from build123d import *

# Parameters (mm, degrees)
F1_DEPTH = 6.35


with BuildPart() as f1:
    # F0 (on Top) → F1 (new body)
    with BuildSketch(Plane.XY):
        with BuildLine():
            ThreePointArc((-3.1267646158, 0.5513329641), (0.2767194832, 3.1629181664), (3.175, 0))
            Line((3.175, 0), (9.525, 0))
            ThreePointArc((9.525, 0), (6.7351920908, 6.7351920908), (0, 9.525))
            ThreePointArc((0, 9.525), (-6.1225519823, 7.2965733207), (-9.3802938474, 1.6539988923))
            Line((-9.3802938474, 1.6539988923), (-3.1267646158, 0.5513329641))
        make_face()
        with BuildLine():
            Line((9.525, 0), (3.175, 0))
            ThreePointArc((3.175, 0), (0, -3.175), (-3.175, 0))
            Line((-3.175, 0), (-9.525, 0))
            ThreePointArc((-9.525, 0), (-7.8202053152, -5.4378317212), (-3.316073212, -8.9291255704))
            Line((-3.316073212, -8.9291255704), (0, -9.525))
            ThreePointArc((0, -9.525), (6.7351920908, -6.7351920908), (9.525, 0))
        make_face()
        with BuildLine():
            ThreePointArc((0, 9.525), (6.7351920908, 6.7351920908), (9.525, 0))
            Line((9.525, 0), (50.1904, 0))
            ThreePointArc((50.1904, 0), (52.9802079092, 6.7351920908), (59.7154, 9.525))
            Line((59.7154, 9.525), (0, 9.525))
        make_face()
        with BuildLine():
            Line((50.1904, 0), (9.525, 0))
            ThreePointArc((9.525, 0), (6.7351920908, -6.7351920908), (0, -9.525))
            Line((0, -9.525), (59.7154, -9.525))
            ThreePointArc((59.7154, -9.525), (52.9802079092, -6.7351920908), (50.1904, 0))
        make_face()
        with BuildLine():
            ThreePointArc((-3.316073212, -8.9291255704), (-7.8202053152, -5.4378317212), (-9.525, 0))
            Line((-9.525, 0), (-40.1437268637, 0))
            ThreePointArc((-40.1437268637, 0), (-42.2877419599, -1.0354554234), (-44.6215756209, -1.5068248214))
            Line((-44.6215756209, -1.5068248214), (-3.316073212, -8.9291255704))
        make_face()
        with BuildLine():
            Line((-35.9452860234, 6.3381237552), (-9.3802938474, 1.6539988923))
            ThreePointArc((-9.3802938474, 1.6539988923), (-6.1225519823, 7.2965733207), (0, 9.525))
            Line((0, 9.525), (-43.6409873472, 17.3669705411))
            ThreePointArc((-43.6409873472, 17.3669705411), (-38.0190290845, 14.1027642346), (-35.8005798708, 7.9921226475))
            ThreePointArc((-35.8005798708, 7.9921226475), (-35.8368253715, 7.1619641978), (-35.9452860234, 6.3381237552))
        make_face()
        with BuildLine():
            ThreePointArc((59.7154, 9.525), (52.9802079092, 6.7351920908), (50.1904, 0))
            ThreePointArc((50.1904, 0), (52.9802079092, -6.7351920908), (59.7154, -9.525))
            ThreePointArc((59.7154, -9.525), (66.4505920908, -6.7351920908), (69.2404, 0))
            ThreePointArc((69.2404, 0), (66.4505920908, 6.7351920908), (59.7154, 9.525))
        make_face()
        with BuildLine():
            ThreePointArc((62.8904, 0), (59.7154, -3.175), (56.5404, 0))
            ThreePointArc((56.5404, 0), (59.7154, 3.175), (62.8904, 0))
        make_face(mode=Mode.SUBTRACT)
        with BuildLine():
            ThreePointArc((-3.316073212, -8.9291255704), (-1.6845925237, -9.3748478937), (0, -9.525))
            Line((0, -9.525), (-3.316073212, -8.9291255704))
        make_face()
        with BuildLine():
            ThreePointArc((-44.6215756209, -1.5068248214), (-42.2877419599, -1.0354554234), (-40.1437268637, 0))
            ThreePointArc((-40.1437268637, 0), (-37.3847371298, 2.7320236406), (-35.9452860234, 6.3381237552))
            ThreePointArc((-35.9452860234, 6.3381237552), (-35.8368253715, 7.1619641978), (-35.8005798708, 7.9921226475))
            ThreePointArc((-35.8005798708, 7.9921226475), (-38.0190290845, 14.1027642346), (-43.6409873472, 17.3669705411))
            ThreePointArc((-43.6409873472, 17.3669705411), (-54.414733052, 10.8404413532), (-49.2925454975, -0.6674852372))
            Line((-49.2925454975, -0.6674852372), (-44.6215756209, -1.5068248214))
        make_face()
        with BuildLine():
            ThreePointArc((-42.1505798708, 7.9921226475), (-42.1626617044, 7.7154031643), (-42.198815255, 7.4407896834))
            ThreePointArc((-42.198815255, 7.4407896834), (-48.4884980373, 8.2688421307), (-42.1505798708, 7.9921226475))
        make_face(mode=Mode.SUBTRACT)
        with BuildLine():
            ThreePointArc((-49.2925454975, -0.6674852372), (-47.0101723945, -1.3827252462), (-44.6215756209, -1.5068248214))
            Line((-44.6215756209, -1.5068248214), (-49.2925454975, -0.6674852372))
        make_face()
        with BuildLine():
            Line((-40.1437268637, 0), (-9.525, 0))
            ThreePointArc((-9.525, 0), (-9.4887544993, 0.8301584497), (-9.3802938474, 1.6539988923))
            Line((-9.3802938474, 1.6539988923), (-35.9452860234, 6.3381237552))
            ThreePointArc((-35.9452860234, 6.3381237552), (-37.3847371298, 2.7320236406), (-40.1437268637, 0))
        make_face()
        with BuildLine():
            Line((-9.525, 0), (-3.175, 0))
            ThreePointArc((-3.175, 0), (-3.1629181664, 0.2767194832), (-3.1267646158, 0.5513329641))
            Line((-3.1267646158, 0.5513329641), (-9.3802938474, 1.6539988923))
            ThreePointArc((-9.3802938474, 1.6539988923), (-9.4887544993, 0.8301584497), (-9.525, 0))
        make_face()
    extrude(amount=F1_DEPTH)


solid = f1.part
Source: CAD feature listing. Evaluate the final solid. Frame: model axes, mm. A direction names the side the tool comes from. Round coordinates to 2 decimals unless told otherwise and drop trailing zeros. Loops run counter-clockwise (first coordinate to the right, second up) from the corner with the lowest first, then second, coordinate; pieces in that order, holes last. Notation, with made-up numbers: M 84,-40 L 131,-40 A27 cw 131,-4 Z; hole C -16.75,-31 d3. An arc over 180 degrees is marked long. Answer as CSV lines item,"result".
Q1. Line query: line 1 along Y through (x, z) = (10.5, 4) (3 decimals); line 2 along Y through (x, z) = (-2.5, 4.5); line 3 along X through (y, z) = (8, 2). Output: solid intervals per line, ascending.
Verdict:
line 1,"y = -9.525 to 9.525"
line 2,"y = -9.19 to -1.96, 1.96 to 9.97"
line 3,"x = -54.85 to -48.5, -42.15 to 64.89"
Q2. Cut plane C-C (x = 34.5). Return the cut outline in (y, z) (3 decimals), plus the area to 3 significant figures.
Verdict:
outline,"M -9.525,0 L 9.525,0 L 9.525,6.35 L -9.525,6.35 Z"
area,"121 mm^2"
Q3. Cut plane D-D (y = 12.25). Return the cut outline in (x, z), plus the area to 3 significant figures.
Verdict:
outline,"M -53.85,0 L -15.16,0 L -15.16,6.35 L -53.85,6.35 Z"
area,"246 mm^2"
Q4. Reachability of faces 5 (the face through (-1.71, -9.37, 3.13)), 6 (the face through (30, 9.525, 3)) from +Z, -Z, +X, -X, +Y, -Y: full face, straight path, thin tool, end or side. Return the list, or none.
Verdict:
face 5,"+Z, -Z, -X, -Y"
face 6,"+Z, -Z, +X, +Y"
Q5. Cut plane A-A (z = 3.5). Return the cut outline in (x, y) (3 decimals).
Verdict:
outline,"M -44.622,-1.507 L -3.316,-8.929 A9.525 ccw 0,-9.525 L 59.715,-9.525 A9.525 ccw 59.715,9.525 L 0,9.525 L -43.641,17.367 A9.525 ccw long Z; hole C -45.326,7.992 d6.35; hole C 0,0 d6.35; hole C 59.715,0 d6.35"
Q6. Contact query for a flat-ended pin moving along its axis: pin 1 (5 mm diameter, centred on x = 59.72, y = 0, fed in from -Z) (1 decimal). Output: stop coordinate, or through.
Verdict:
pin 1,"passes through"
Q7. Cut plane B-B (x = -46.5). Return the cut outline in (y, z).
Verdict:
outline,"M -1.46,0 L 5.04,0 L 5.04,6.35 L -1.46,6.35 Z; M 10.94,0 L 17.44,0 L 17.44,6.35 L 10.94,6.35 Z"
Q8. Pull-direction query (X, two-part tool) for faces 1 (the face through (-24.258, -5.166, 3.131)), 2 (the face through (56.783, -1.216, 3.131)), 3 (the face through (29, -9.525, 3)), 4 (the face through (-21.52, 13.39, 3.13)); classes: +X half, -X half, draft (parallel to the pull), parting line (faces both ways), or undercut.
Verdict:
face 1,"-X half"
face 2,"undercut"
face 3,"draft"
face 4,"+X half"
